Source: CAD feature listing. Evaluate the final solid. Frame: model axes, mm. Coordinates: 2 decimals unless noted, no trailing zeros. Loops run counter-clockwise (first coordinate to the right, second up) from the corner with the lowest first, then second, coordinate; pieces in that order, holes last. Notation, with made-up numbers: (-5, 42) - (30, 42) arc R15 cw to (30, 58) - close; hole circle Ø10 at (27, 48). An arc over 180 degrees is marked (long way). Use one line per item in the form item = value. Start each with the question number.
from build123d import *

# Parameters (mm, degrees)
F0_W     = 76.2
F0_H     = 19.05
F1_DEPTH = 625.475
F2_SIZE2 = 19.04999
F2_SIZE  = 19.04999


# Not quite as in the source:
# - a fillet or chamfer is up to 0.001 mm smaller than in the source, because OpenCascade refuses the exact size


with BuildPart() as f1:
    # F0 (on Top) → F1 (new body, symmetric)
    with BuildSketch(Plane.XY):
        Rectangle(F0_W, F0_H)
    extrude(amount=F1_DEPTH, both=True)

    # F2 (size 19.05 and 19.05 in the source; OpenCascade refuses exactly that, so slightly less here)
    f2_edges = [f1.edges().sort_by_distance(p)[0] for p in [
        (-38.1, 9.525, 0),
    ]]
    chamfer(f2_edges, length=F2_SIZE, length2=F2_SIZE2)


solid = f1.part
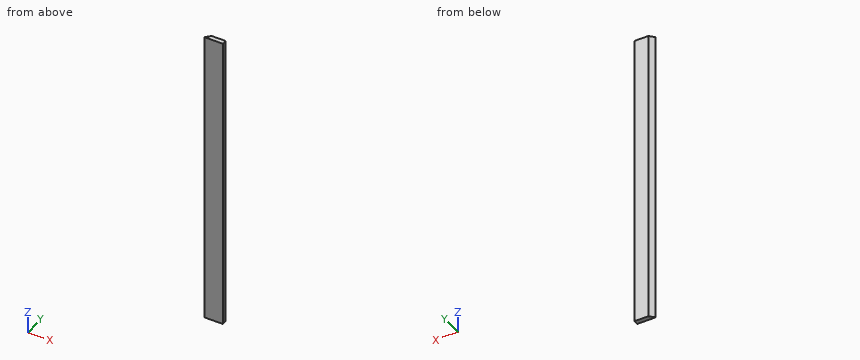
(1) Cut plane B-B, the plane y = -3.5. Output: boundary loops of the cut face in (x, z) (3 decimals).
(2) Contact query for a flat-ended pin moving along its axis: pin 1 (3 mm diameter, centred on y = -0.5, z = -301, fed in from -X) (3 decimals). Output: stop coordinate, or through.
(3) Material intervals for line 1 (X direction, y = 0, z = -271); line 2 (X direction, y = -6.75, z = -127); line 3 (Y direction, x = -21.5, z = -401.5) (3 decimals), sorted ascending.
Recorded:
q1.outline = (-32.075, -625.475) - (38.1, -625.475) - (38.1, 625.475) - (-32.075, 625.475) - close
q2.pin_1 = -30.575
q3.line_1 = -28.58 to 38.1
q3.line_2 = -35.33 to 38.1
q3.line_3 = -9.525 to 7.075
